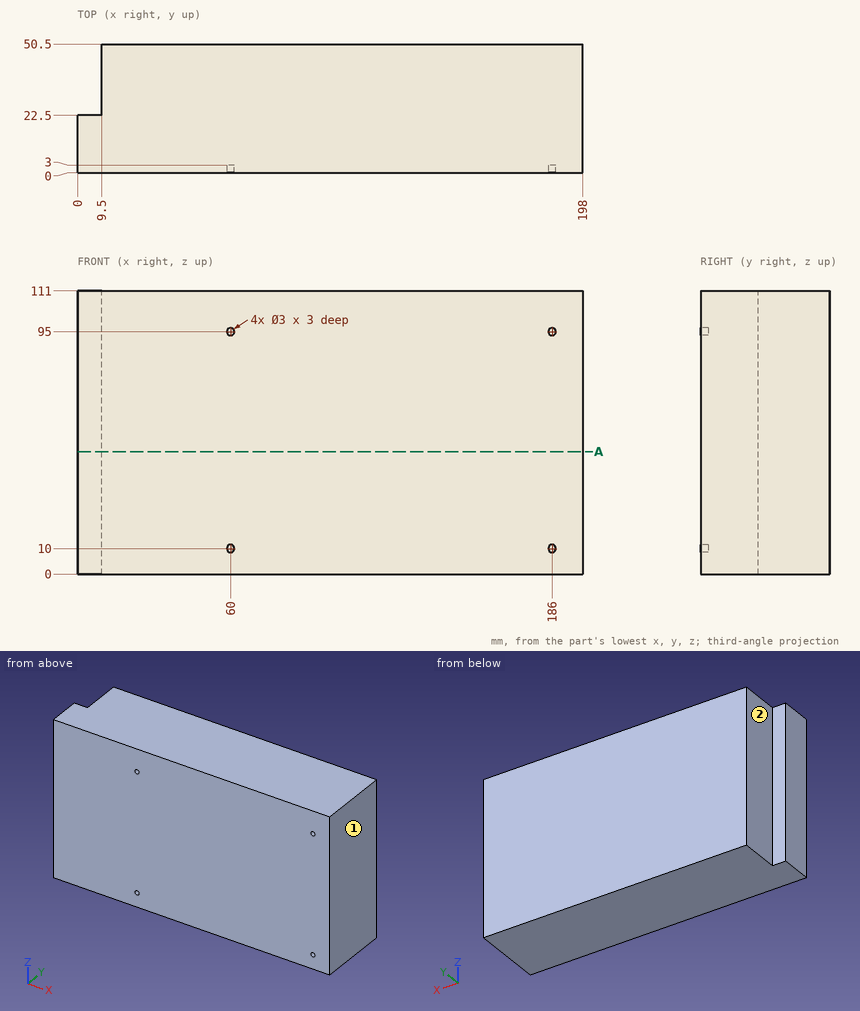
Input: dimensioned drawing with shaded views. Units: mm. Origin: part minimum x, y, z. A direction names the side the tool comes from. Give positions to 0.01 mm unless a question says otherwise; leave off trailing zeros. Write each loop counter-clockwise with the first axis right and the second up, starting at its lowest first coordinate (ties: lowest second). Pieces come first, ordered by that corner, then holes.
Q1. First-contact query: P1, Ø4, axis at y = 26.5, z = 67.5, coming from the -X side; P2, Ø1.5, axis at x = 60, z = 9.5, coming from the -Y side. Flat tips, straight axial feed; report the tip coordinate or a pass-through.
Q2. Section A-A, the plane z = 48. Output: boundary loops of the cut face in (x, y).
Q3. Material intervals for probe 1 along Z at (x, y) = (186, 1); probe 2 along X at (y, z) = (1.75, 95); probe 3 along X at (y, z) = (26, 45), sorted ascending.
Q4. Set-up query: the marked faces 1 and 2. Return all of +Z, -Z, +X, -X, +Y, -Y with unobstructed straight access to the full face (end or side cutting, diameter ignored); none if empty.
Filled in:
1. P1: stops at x = 9.5
1. P2: stops at y = 3
2. outline: (0, 0) - (198, 0) - (198, 50.5) - (9.5, 50.5) - (9.5, 22.5) - (0, 22.5) - close
3. probe 1: z = 0 to 8.5, 11.5 to 93.5, 96.5 to 111
3. probe 2: x = 0 to 58.5, 61.5 to 184.5, 187.5 to 198
3. probe 3: x = 9.5 to 198
4. face 1: +Z, -Z, +X, +Y, -Y
4. face 2: +Z, -Z, -X, +Y
